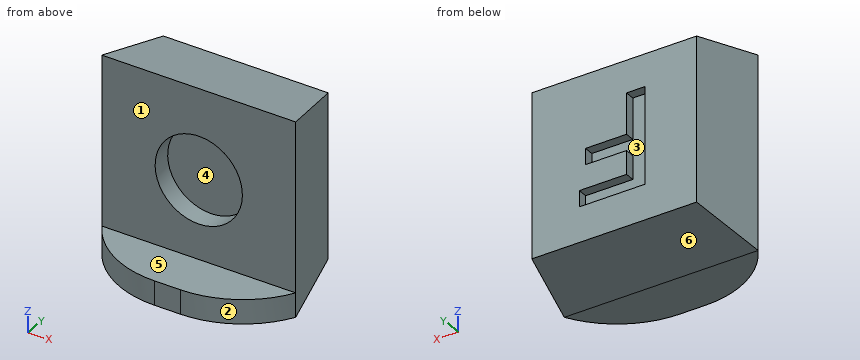
```python
from build123d import *

# Parameters (mm, degrees)
SKETCH1_W               = 8
SKETCH1_H               = 8
BOSS_EXTRUDE1_DEPTH     = 3
CUT_EXTRUDE1_DEPTH      = 12.704699911
CUT_EXTRUDE1_DEPTH_BACK = 12.704699911
CUT_EXTRUDE2_DEPTH      = 11
SKETCH4_R               = 1.8
CUT_EXTRUDE3_DEPTH      = 0.8
SKETCH5_W               = 8
SKETCH5_H               = 1
BOSS_EXTRUDE2_DEPTH     = 2
FILLET1_R               = 4
CUT_EXTRUDE4_DEPTH      = 0.4


with BuildPart() as part:
    # Sketch1 → Boss-Extrude1 (new body)
    with BuildSketch(Plane(origin=(0, 0, 0), x_dir=(1, 0, 0), z_dir=(0, 1, 0))):
        with Locations((4, 4)):
            Rectangle(SKETCH1_W, SKETCH1_H)
    extrude(amount=BOSS_EXTRUDE1_DEPTH)

    # Sketch2 → Cut-Extrude1 (cut, two sides: drawn at the far end of the back side and taken through both)
    with BuildSketch(Plane.XY.offset(-CUT_EXTRUDE1_DEPTH_BACK)):
        Polygon((0, 0), (0.6, 3), (0, 3), align=None)
        Polygon((8, 0), (7.4, 3), (8, 3), align=None)
    extrude(amount=CUT_EXTRUDE1_DEPTH + CUT_EXTRUDE1_DEPTH_BACK, mode=Mode.SUBTRACT)

    # Sketch3 → Cut-Extrude2 (cut)
    with BuildSketch(Plane(origin=(0, 0, 0), x_dir=(0, 0, -1), z_dir=(1, 0, 0))):
        Polygon((0, 0), (0.6, 3), (0, 3), align=None)
        Polygon((8, 3), (7.4, 3), (8, 0), align=None)
    extrude(amount=CUT_EXTRUDE2_DEPTH, mode=Mode.SUBTRACT)

    # Sketch4 → Cut-Extrude3 (cut)
    with BuildSketch(Plane.XZ):
        with Locations(Location((4, -3.75, 0), (0, 0, 270))):
            Circle(SKETCH4_R)
    extrude(amount=-CUT_EXTRUDE3_DEPTH, mode=Mode.SUBTRACT)

    # Sketch5 → Boss-Extrude2 (add)
    with BuildSketch(Plane.XZ):
        with Locations((4, -7.5)):
            Rectangle(SKETCH5_W, SKETCH5_H)
    extrude(amount=BOSS_EXTRUDE2_DEPTH)

    # Fillet1
    # the kernel refuses this fillet: 4 mm, written as the material it takes off along each edge
    with BuildSketch(Plane(origin=(8, -2, -16.660254038), x_dir=(0, 1, 0), z_dir=(0, 0, 1)), Plane(origin=(0, -2, 1.660254038), x_dir=(0, 1, 0), z_dir=(0, 0, -1))) as fillet1_piece_1:
        with BuildLine():
            CenterArc((4, 3.464101615), FILLET1_R, 180, 60)
            Line((0, 3.464101615), (-0.08, 3.464101615))
            Line((-0.08, 3.464101615), (-0.08, 0))
            Line((-0.08, 0), (0, -0.08))
            ThreePointArc((0, -0.08), (1, -0.08), (1.96, -0.069282032))
            Line((1.96, -0.069282032), (2, 0))
        make_face()
    extrude(amount=18.320508076, mode=Mode.SUBTRACT)

    # Sketch6 → Cut-Extrude4 (cut)
    with BuildSketch(Plane(origin=(0, 3, 0), x_dir=(1, 0, 0), z_dir=(0, 1, 0))):
        Polygon((2.721575188, 1.941169366), (2.721575188, 5.941169366), (5.439523906, 5.941169366), (5.439523906, 5.2745027), (3.490805957, 5.2745027), (3.490805957, 4.300143725), (5.18311365, 4.300143725), (5.18311365, 3.633477059), (3.490805957, 3.633477059), (3.490805957, 1.941169366), align=None)
    extrude(amount=-CUT_EXTRUDE4_DEPTH, mode=Mode.SUBTRACT)


solid = part.part
```
CAD build for the part. Positions are in the model's coordinates, mm. Face numbers are marked on the shaded views. A direction names the side the tool comes from. Coordinates: 2 decimals unless noted, no trailing zeros. Write each loop counter-clockwise with the first axis right and the second up, starting at its lowest first coordinate (ties: lowest second). Pieces come first, ordered by that corner, then holes. Notation, with made-up numbers: (53.25, 47.25) -> (65.25, 47.25) arc R18 ccw to (65.25, 51.25) -> close; hole circle Ø11 at (-13, 31.25). An arc over 180 degrees is marked (long way). Return JSON: item names as keys, results as strings. Group by question number.
Q1. Drill centre lines: line 1 (Z direction, x = 4.25, y = -1.7); line 2 (Y direction, x = 3.75, z = -2.25); line 3 (Y direction, x = 3.25, z = -5.25). Where is each one in solid material? Low to high.
Q2. Cut at D-D, the plane y = 1.85. Give the cut face in (x, z), then the cut area to 3 significant figures.
Q3. Pull direction Z, two halves, no side cores. Call the marked faces 3, 4, 5 and 6: released by +Z, released by -Z, zero draft, split by the parting line, or undercut.
Q4. Cut at C-C, the plane z = -3.75. Give the cut face in (x, y), then the cut area to 3 significant figures.
Q5. Which spindle directions (+Z, -Z, +X, -X, +Y, -Y) get a long thin tool onto all of the face, cutting with end or side? Do the marked faces 1 and 2. Say none if no direction does.
Q6. Flat gauge pins, fed straight in: pin 1 (0.6 mm diameter, centred on x = 4, y = -1, fed in from +Z); pin 2 (3 mm diameter, centred on x = 4.5, z = -3.5, fed in from -Y). Where does each tip first touch, or does it go through?
Q7. Cut at A-A, the plane x = 4. Give the cut face in (y, z), then the cut area to 3 significant figures.
Q8. Cut at B-B, the plane y = 0.6. Give the cut face in (x, z), then the cut area to 3 significant figures.
Returned:
{
 "1": {"line 1": "z = -8 to -7", "line 2": "y = 0.8 to 3", "line 3": "y = 0.8 to 2.6"},
 "2": {"outline": "(0.37, -7.63) -> (7.63, -7.63) -> (7.63, -0.37) -> (0.37, -0.37) -> close", "area": "52.7 mm2"},
 "3": {"face 3": "undercut", "face 4": "undercut", "face 5": "released by +Z", "face 6": "released by -Z"},
 "4": {"outline": "(0, 0) -> (2.2, 0) -> (2.2, 0.8) -> (5.8, 0.8) -> (5.8, 0) -> (8, 0) -> (7.4, 3) -> (5.18, 3) -> (5.18, 2.6) -> (2.72, 2.6) -> (2.72, 3) -> (0.6, 3) -> close", "area": "18.3 mm2"},
 "5": {"face 1": "+Z, +X, -X, -Y", "face 2": "+Z, -Z, +X, -Y"},
 "6": {"pin 1": "stops at z = -7", "pin 2": "stops at y = 0"},
 "7": {"outline": "(-2, -8) -> (0, -8) -> (3, -7.4) -> (3, -5.94) -> (2.6, -5.94) -> (2.6, -5.27) -> (3, -5.27) -> (3, -4.3) -> (2.6, -4.3) -> (2.6, -3.63) -> (3, -3.63) -> (3, -0.6) -> (0, 0) -> (0, -1.95) -> (0.8, -1.95) -> (0.8, -5.55) -> (0, -5.55) -> (0, -7) -> (-2, -7) -> close", "area": "20.8 mm2"},
 "8": {"outline": "(0.12, -7.88) -> (7.88, -7.88) -> (7.88, -0.12) -> (0.12, -0.12) -> close; hole circle Ø3.6 at (4, -3.75)", "area": "50.0 mm2"}
}
